Check sheet for the modelled part. Datum: model origin and axes. Units: mm. A direction names the side the tool comes from. Give positions to 0.01 mm unless a question says otherwise; leave off trailing zeros. Order: outer loops, then holes, each group sorted by start corner. A loop starts at its lowest first (then second) coordinate and runs counter-clockwise, first axis right, second up.
```python
from build123d import *

# Parameters (mm, degrees)
F1_DEPTH = 3
F3_DEPTH = 16.5
F5_W     = 20
F5_H     = 8.7
F6_DEPTH = 25
F7_W     = 20
F7_H     = 8.5
F8_DEPTH = 25


with BuildPart() as f1:
    # F0 (on Top) → F1 (new body)
    with BuildSketch(Plane.XY):
        Polygon((0, 36), (0, 0), (36, 0), (36, 3), (3, 36), align=None)
    extrude(amount=F1_DEPTH)

    # F2 (on face) → F3 (join)
    with BuildSketch(Plane.XY.offset(3)):
        Polygon((3, 3), (3, 36), (0, 36), (0, 0), (36, 0), (36, 3), align=None)
    extrude(amount=F3_DEPTH)

    # F4: F1 across face


with BuildPart() as f1_1:
    add(f1.part)
    add(f1.part.mirror(Plane(origin=(10.1086956522, 10.1086956522, 19.5), x_dir=(1, 0, 0), z_dir=(0, 0, 1))))

    # F5 (on face) → F6 (cut)
    with BuildSketch(Plane.XZ):
        with Locations((18, 19.5)):
            Rectangle(F5_W, F5_H)
    extrude(amount=-F6_DEPTH, mode=Mode.SUBTRACT)

    # F7 (on face) → F8 (cut)
    with BuildSketch(Plane(origin=(0, 0, 0), x_dir=(0, -1, 0), z_dir=(-1, 0, 0))):
        with Locations((-18, 19.5)):
            Rectangle(F7_W, F7_H)
    extrude(amount=-F8_DEPTH, mode=Mode.SUBTRACT)


solid = f1_1.part
```
(1) Sectioned sample at A-A (y = 26). Enter the section's corners in (x, z), plus the area to 4 significant figures.
(2) Thickness scan on L1, parallel to Z at x = 14, y = 17.5; L2, parallel to X at y = 5, z = 30.5. Record the ranges inside material, lowest first.
(3) Sectioned sample at B-B (z = 21.5). Enter the section's corners in (x, y), plus the area to 3 significant figures.
(4) Sectioned sample at C-C (x = 20.5). Enter the section's corners in (y, z), plus the area to 3 significant figures.
(5) Tool access check on faces 4 (the face through (20, 3, 12)), 5 (the face through (18, 1, 15.15)), 6 (the face through (1, 28, 19)). Record the directions out of +Z, -Z, +X, -X, +Y, -Y that give a thin tool (end or side, any length) a straight path to the whole face; none if there is none.
(6) Release check for a two-part mould opening along Z. For faces 1 (the face through (14, 14, 0)), 2 (the face through (36, 1, 20)), 3 (the face through (12, 12, 36)) record: released by +Z, released by -Z, zero draft, split by the parting line, or undercut.
(7) Sectioned sample at D-D (y = 4). Enter the section's corners in (x, z), plus the area to 3 significant figures.
(8) Go/stop test with a flat-tipped pin: P1, Ø4, axis at x = 31, z = 20.5, coming from the +Y side. Record where the tip stops, or that it passes through.
Values follow:
1. outline: (0, 0) - (13, 0) - (13, 3) - (3, 3) - (3, 15.25) - (0, 15.25) - close; (0, 23.75) - (3, 23.75) - (3, 36) - (13, 36) - (13, 39) - (0, 39) - close
1. area: 151.5 mm2
2. L1: z = 0 to 3, 36 to 39
2. L2: x = 0 to 3
3. outline: (0, 0) - (8, 0) - (8, 3) - (3, 3) - (3, 8) - (0, 8) - close; (0, 28) - (3, 28) - (3, 36) - (0, 36) - close; (28, 0) - (36, 0) - (36, 3) - (28, 3) - close
3. area: 87.0 mm2
4. outline: (0, 0) - (18.5, 0) - (18.5, 3) - (3, 3) - (3, 15.15) - (0, 15.15) - close; (0, 23.85) - (3, 23.85) - (3, 36) - (18.5, 36) - (18.5, 39) - (0, 39) - close
4. area: 184 mm2
5. face 4: +X, +Y
5. face 5: +Y, -Y
5. face 6: +X, -X
6. face 1: released by -Z
6. face 2: zero draft
6. face 3: undercut
7. outline: (0, 0) - (35, 0) - (35, 3) - (3, 3) - (3, 36) - (35, 36) - (35, 39) - (0, 39) - close
7. area: 309 mm2
8. P1: stops at y = 3
